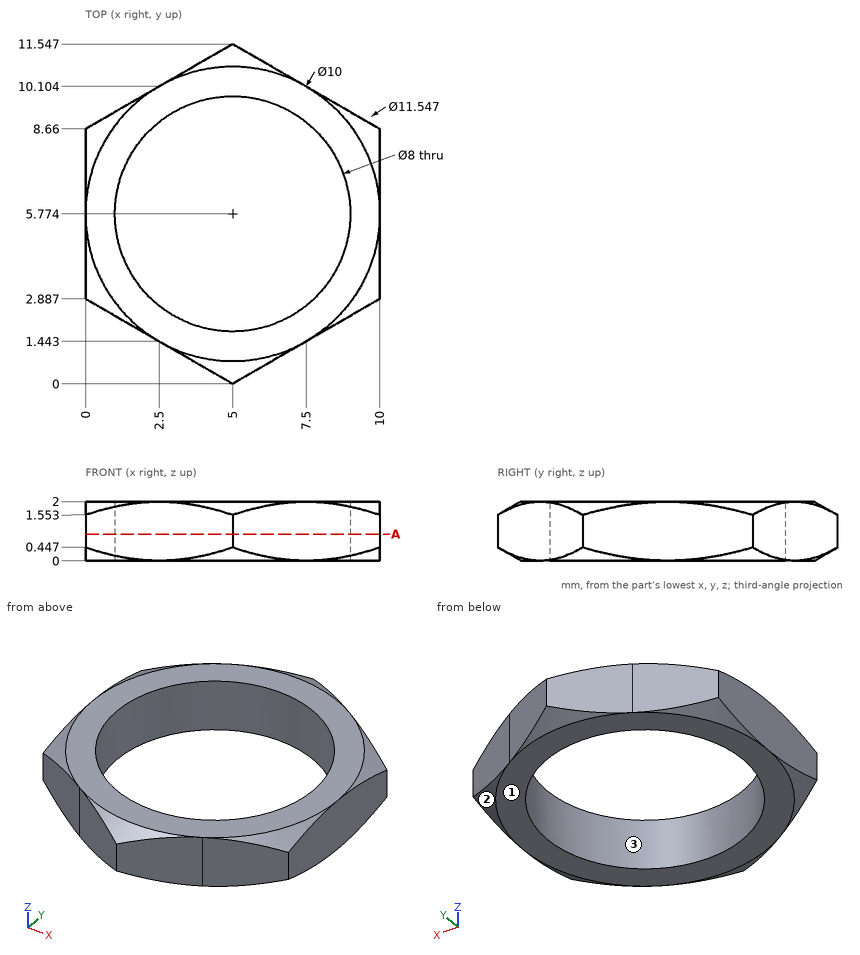
Here's the drawing with two shaded views (mm, measured from the low corner). I have some questions. Round coordinates to 2 decimals unless told otherwise and drop trailing zeros. Loops run counter-clockwise (first coordinate to the right, second up) from the corner with the lowest first, then second, coordinate; pieces in that order, holes last.
Item 1: Please list where these lines run through material, in increasing order: L1, parallel to Y at x = 5.5, z = 1.65 (1 decimal); L2, parallel to X at y = 9, z = 0.75 (1 decimal); L3, parallel to X at y = 2.75, z = 1.3 (1 decimal).
Item 2: If we mould it in two halves opening along Y, with no side actions, what happens to the marked faces 1, 2 and 3? For each: +Y half, -Y half, draft (parallel to the pull), parting line (faces both ways), or undercut.
Item 3: Will this pin go through, and if not, where does the flat tip stop? pin 1 Ø1 at (x, z) = (3, 0) entering from +Y.
Item 4: Suppose I cut it at A-A, the plane z = 0.9. Write out the boundary of the cut face in (x, y).
Reported:
1. L1: y = 0.3 to 1.8, 9.7 to 11.3
1. L2: x = 0.6 to 2.6, 7.4 to 9.4
1. L3: x = 0.2 to 2.4, 7.6 to 9.8
2. face 1: draft
2. face 2: +Y half
2. face 3: undercut
3. pin 1: stops at y = 10.68
4. outline: (0, 2.89) - (5, 0) - (10, 2.89) - (10, 8.66) - (5, 11.55) - (0, 8.66) - close; hole circle Ø8 at (5, 5.77)
